Geometry check sheet. Reference: the model listing, model coordinates, mm. Face numbers are marked on the shaded views. A direction names the side the tool comes from. Give positions to 0.01 mm unless a question says otherwise; leave off trailing zeros. Write each loop counter-clockwise with the first axis right and the second up, starting at its lowest first coordinate (ties: lowest second). Pieces come first, ordered by that corner, then holes. Notation, with made-up numbers: (21, 30.25) -> (63, 30.25) arc R20 ccw to (63, 49.25) -> close; hole circle Ø5 at (57.25, -22.5). An arc over 180 degrees is marked (long way). One line per item, written item: value.
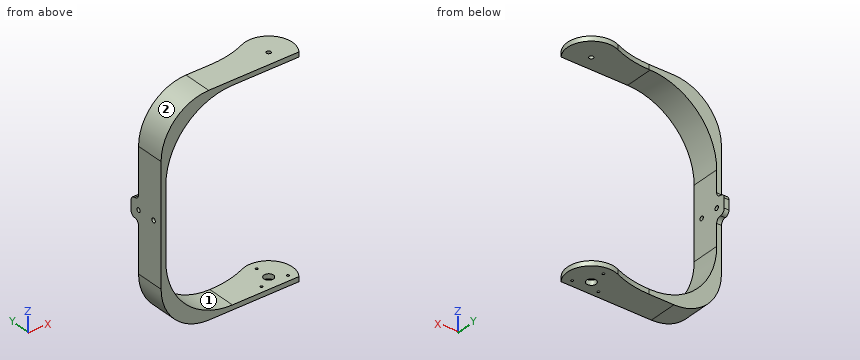
from build123d import *

# Parameters (mm, degrees)
SKETCH1_W           = 125
SKETCH1_H           = 30
BOSS_EXTRUDE1_DEPTH = 112.5
BOSS_EXTRUDE2_DEPTH = 112.5
CUT_EXTRUDE2_START  = 5
SKETCH4_W           = 215
SKETCH4_H           = 59.703545047
CUT_EXTRUDE2_DEPTH  = 160
SKETCH5_R           = 1.25
SKETCH5_R_2         = 5
CUT_EXTRUDE3_DEPTH  = 10
FILLET1_R           = 100
FILLET2_R           = 70
FILLET3_R           = 50
SKETCH7_W           = 20
SKETCH7_H           = 10
BOSS_EXTRUDE3_DEPTH = 5
SKETCH6_R           = 2.25
CUT_EXTRUDE4_DEPTH  = 10
FILLET4_R           = 5
FILLET5_R           = 5
SKETCH8_R           = 2.25
CUT_EXTRUDE5_DEPTH  = 5


with BuildPart() as part:
    # Sketch1 → Boss-Extrude1 (new, symmetric)
    with BuildSketch(Plane.XY):
        with Locations((62.5, 15)):
            Rectangle(SKETCH1_W, SKETCH1_H)
    extrude(amount=BOSS_EXTRUDE1_DEPTH, both=True)

    # Sketch2 → Boss-Extrude2 (add, symmetric)
    with BuildSketch(Plane.XY):
        with BuildLine():
            Line((105, 0), (145, 0))
            ThreePointArc((145, 0), (125, 40), (105, 0))
        make_face()
    extrude(amount=BOSS_EXTRUDE2_DEPTH, both=True)

    # Sketch4 → Cut-Extrude2 (cut)
    with BuildSketch(Plane(origin=(0, 0, 0), x_dir=(0, 0, -1), z_dir=(1, 0, 0)).offset(CUT_EXTRUDE2_START)):
        with Locations((0, 25.910589708)):
            Rectangle(SKETCH4_W, SKETCH4_H)
    extrude(amount=CUT_EXTRUDE2_DEPTH, mode=Mode.SUBTRACT)

    # Sketch5 → Cut-Extrude3 (cut)
    with BuildSketch(Plane(origin=(0, 0, -112.5), x_dir=(-1, 0, 0), z_dir=(0, 0, -1))):
        with Locations((-138.856406461, 7)):
            Circle(SKETCH5_R)
        with Locations((-125, 31)):
            Circle(SKETCH5_R)
        with Locations((-111.143593539, 7)):
            Circle(SKETCH5_R)
        with Locations((-125.004149617, 15)):
            Circle(SKETCH5_R_2)
    extrude(amount=-CUT_EXTRUDE3_DEPTH, mode=Mode.SUBTRACT)

    # Fillet1
    fillet1_edges = [part.edges().sort_by_distance(p)[0] for p in [
        (105, 30, -110),
        (105, 30, 110),
    ]]
    fillet(fillet1_edges, radius=FILLET1_R)

    # Fillet2
    fillet2_edges = [part.edges().sort_by_distance(p)[0] for p in [
        (5, 15, 107.5),
        (5, 15, -107.5),
    ]]
    fillet(fillet2_edges, radius=FILLET2_R)

    # Fillet3
    fillet3_edges = [part.edges().sort_by_distance(p)[0] for p in [
        (0, 15, 112.5),
        (0, 15, -112.5),
    ]]
    fillet(fillet3_edges, radius=FILLET3_R)

    # Sketch7 → Boss-Extrude3 (add)
    with BuildSketch(Plane.ZY):
        with Locations((0, 35)):
            Rectangle(SKETCH7_W, SKETCH7_H)
    extrude(amount=-BOSS_EXTRUDE3_DEPTH)

    # Sketch6 → Cut-Extrude4 (cut)
    with BuildSketch(Plane.ZY):
        with Locations((0, 10)):
            Circle(SKETCH6_R)
        with Locations((0, 30)):
            Circle(SKETCH6_R)
    extrude(amount=-CUT_EXTRUDE4_DEPTH, mode=Mode.SUBTRACT)

    # Fillet4
    fillet4_edges = [part.edges().sort_by_distance(p)[0] for p in [
        (2.5, 30, 10),
        (2.5, 30, -10),
    ]]
    fillet(fillet4_edges, radius=FILLET4_R)

    # Fillet5
    fillet5_edges = [part.edges().sort_by_distance(p)[0] for p in [
        (2.5, 40, 10),
        (2.5, 40, -10),
    ]]
    fillet(fillet5_edges, radius=FILLET5_R - 0.0001)  # a hair under: the kernel refuses the full size

    # Sketch8 → Cut-Extrude5 (cut)
    with BuildSketch(Plane(origin=(0, 0, 107.5), x_dir=(-1, 0, 0), z_dir=(0, 0, -1))):
        with Locations(Location((-125, 15, 0), (0, 0, 90))):
            Circle(SKETCH8_R)
    extrude(amount=-CUT_EXTRUDE5_DEPTH, mode=Mode.SUBTRACT)


solid = part.part
1) Sectioned sample at B-B on z = 0. Record the cut outline in (x, y).
Verdict:
outline: (0, 0) -> (5, 0) -> (5, 7.75) -> (0, 7.75) -> close; (0, 12.25) -> (5, 12.25) -> (5, 27.75) -> (0, 27.75) -> close; (0, 32.25) -> (5, 32.25) -> (5, 40) -> (0, 40) -> close
2) Sectioned sample at C-C on x = 39.5. Record the cut outline in (y, z).
Verdict:
outline: (0, -111.39) -> (30, -111.39) -> (30, -97.83) -> (0, -97.83) -> close; (0, 97.83) -> (30, 97.83) -> (30, 111.39) -> (0, 111.39) -> close
3) Sectioned sample at D-D on z = 26. Record the cut outline in (x, y), plus the area to 3 significant figures.
Verdict:
outline: (0, 0) -> (5, 0) -> (5, 30) -> (0, 30) -> close
area: 150 mm^2
4) Sectioned sample at A-A on y = 15. Record the cut outline in (x, z).
Verdict:
outline: (0, -62.5) arc R50 ccw to (50, -112.5) -> (120, -112.5) -> (120, -107.5) -> (75, -107.5) arc R70 cw to (5, -37.5) -> (5, 37.5) arc R70 cw to (75, 107.5) -> (122.75, 107.5) -> (122.75, 112.5) -> (50, 112.5) arc R50 ccw to (0, 62.5) -> close; (127.25, 107.5) -> (150, 107.5) -> (150, 112.5) -> (127.25, 112.5) -> close; (130, -112.5) -> (150, -112.5) -> (150, -107.5) -> (130, -107.5) -> close
5) Scan lines: probe 1 along Y at (x, z) = (1, 0); probe 2 along Z at (x, y) = (80.5, 23.5); probe 3 along Z at (x, y) = (68, 10.5). Record each from-to range of solid material in increasing order.
Verdict:
probe 1: 0 to 7.75, 12.25 to 27.75, 32.25 to 40
probe 2: -112.5 to -107.5, 107.5 to 112.5
probe 3: -112.5 to -107.15, 107.15 to 112.5
6) Depth check by flat-ended pin: pin 1 Ø3 at (y, z) = (16, -89) entering from -X; pin 2 Ø4 at (y, z) = (6.5, 83.5) entering from -X. Enter the tip coordinate at first touch or a pass-through.
Verdict:
pin 1: x = 6.7
pin 2: x = 3.75
7) Tool access check on the marked faces 1 and 2. Record the directions out of +Z, -Z, +X, -X, +Y, -Y that give a thin tool (end or side, any length) a straight path to the whole face; none if there is none.
Verdict:
face 1: +X, +Y, -Y
face 2: +Z, -X, +Y, -Y
